Geometry: see drawing. Coordinates: mm, zero at the bounding-box minimum. A direction names the side the tool comes from. Give positions to 0.01 mm unless a question says otherwise; leave off trailing zeros. Write each loop counter-clockwise with the first axis right and the second up, starting at its lowest first coordinate (ties: lowest second). Pieces come first, ordered by that corner, then holes. Notation, with made-up numbers: (28.5, 84.5) - (39.5, 84.5) arc R25 ccw to (39.5, 118.5) - close; hole circle Ø2 at (56, 8.5). An arc over 180 degrees is marked (long way). Return JSON: item names as keys, results as strings.
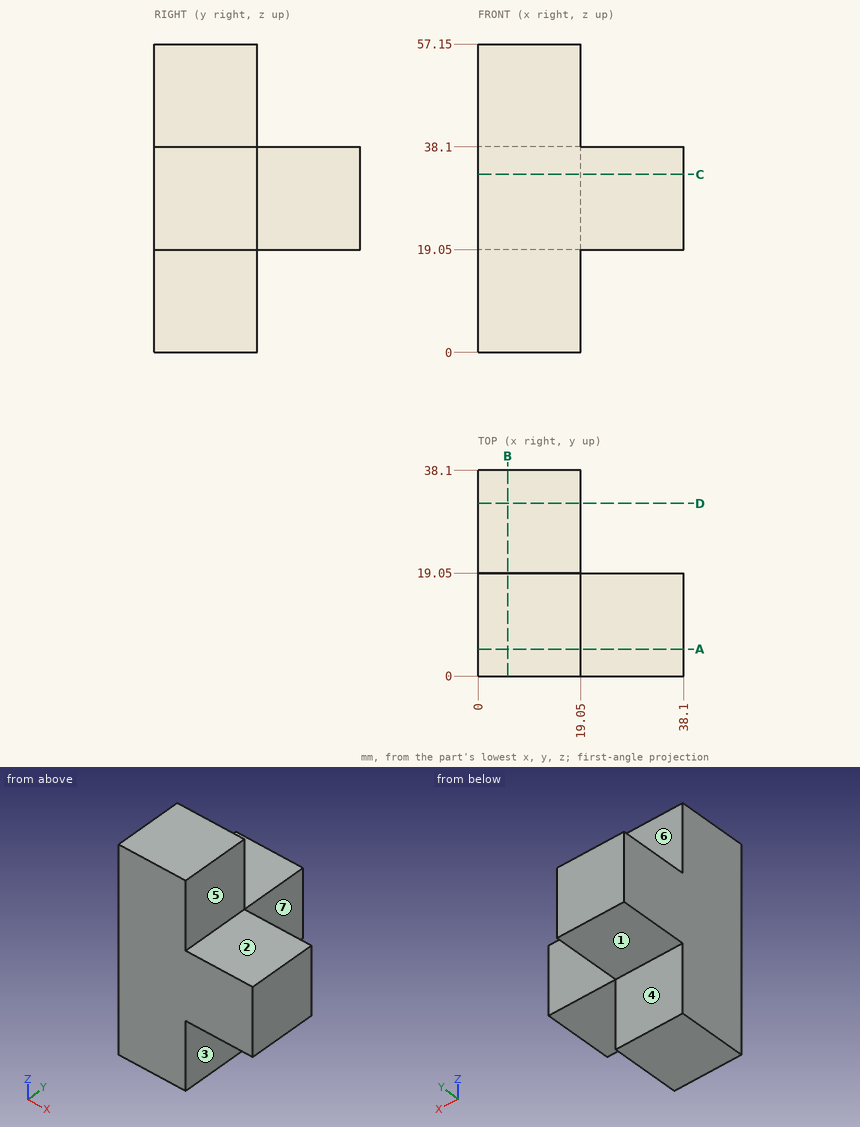
Q1. Mould query, pull axis Z, two halves, no side actions, for the marked faces 1, 2 and 3. Classes: pulls with the +Z half, pulls with the -Z half, needs draft (parallel to the pull), parting line crosses it, or undercut.
Answer key:
{"face 1": "pulls with the -Z half", "face 2": "pulls with the +Z half", "face 3": "needs draft"}
Q2. Section query D-D, the plane y = 32. Return the cut outline in (x, z).
Answer key:
{"outline": "(0, 19.05) - (19.05, 19.05) - (19.05, 38.1) - (0, 38.1) - close"}
Q3. Pin query (flat end, axial travel): P1, Ø9.5, axis at x = 30.5, y = 8, coming from the +Z side; P2, Ø15, axis at x = 11.5, z = 10.5, coming from the +Y side; P3, Ø9.5, axis at y = 31.5, z = 26, coming from the +X side. Return the tip coordinate at first contact, or that it passes through.
Answer key:
{"P1": "stops at z = 38.1", "P2": "stops at y = 19.05", "P3": "stops at x = 19.05"}
Q4. Section query A-A, the plane y = 5. Return the cut outline in (x, z).
Answer key:
{"outline": "(0, 0) - (19.05, 0) - (19.05, 19.05) - (38.1, 19.05) - (38.1, 38.1) - (19.05, 38.1) - (19.05, 57.15) - (0, 57.15) - close"}
Q5. Material intervals for probe 1 along Z at (x, y) = (35, 2); probe 2 along Y at (x, z) = (18.5, 47), sorted ascending. Write a range as [from, to].
Answer key:
{"probe 1": "z = [19.05, 38.1]", "probe 2": "y = [0, 19.05]"}
Q6. Set-up query: the marked faces 4, 5, 6 and 7. Return all of +Z, -Z, +X, -X, +Y, -Y with unobstructed straight access to the full face (end or side cutting, diameter ignored); none if empty.
Answer key:
{"face 4": "-Z, +X, -X, +Y", "face 5": "+Z, +X, +Y, -Y", "face 6": "+Z, +X, -X, +Y", "face 7": "+Z, -Z, +X, +Y"}
Q7. Section query C-C, the plane z = 33. Return the cut outline in (x, y).
Answer key:
{"outline": "(0, 0) - (38.1, 0) - (38.1, 19.05) - (19.05, 19.05) - (19.05, 38.1) - (0, 38.1) - close"}
